Could you check a few things on this model? Use its own coordinates, in mm. Face numbers are marked on the shaded views. A direction names the side the tool comes from. Give positions to 0.01 mm unless a question says otherwise; leave off trailing zeros. Write each loop counter-clockwise with the first axis right and the second up, starting at its lowest first coordinate (ties: lowest second). Pieces come first, ordered by that corner, then holes. Notation, with made-up numbers: M -11,9 L -7,9 A11 ccw -7,24 Z; hole C -24,64 d9. An arc over 180 degrees is marked long. Answer as a JSON object with one key per item and string values. Group by question number.
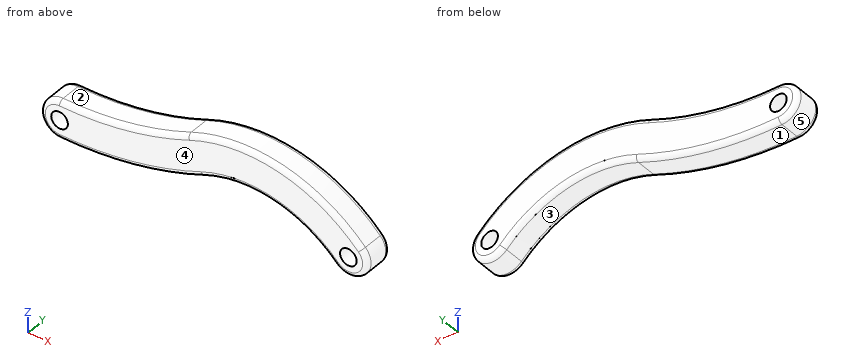
```python
from build123d import *

# Parameters (mm, degrees)
SKETCH1_R           = 1.75
BOSS_EXTRUDE1_DEPTH = 6
FILLET1_R           = 1


with BuildPart() as part:
    # Sketch1 → Boss-Extrude1 (new body)
    with BuildSketch(Plane(origin=(0, 0, 0), x_dir=(1, 0, 0), z_dir=(0, 1, 0))):
        with BuildLine():
            ThreePointArc((-30.4, 4), (-34.4, 0), (-30.4, -4))
            ThreePointArc((-30.4, -4), (-16.617055958, -5.436924168), (-3.426888285, -9.685897488))
            ThreePointArc((-3.426888285, -9.685897488), (15.962258381, -11.93115149), (33.228427125, -2.828427125))
            ThreePointArc((33.228427125, -2.828427125), (33.228427125, 2.828427125), (27.571572875, 2.828427125))
            ThreePointArc((27.571572875, 2.828427125), (14.491142009, -4.067576182), (-0.197605466, -2.366626181))
            ThreePointArc((-0.197605466, -2.366626181), (-14.966930275, 2.391043974), (-30.4, 4))
        make_face()
        with Locations(Location((-30.4, 0, 0), (0, 0, 270))):
            Circle(SKETCH1_R, mode=Mode.SUBTRACT)
        with Locations(Location((30.4, 0, 0), (0, 0, 270))):
            Circle(SKETCH1_R, mode=Mode.SUBTRACT)
    extrude(amount=BOSS_EXTRUDE1_DEPTH)

    # Fillet1
    fillet1_edges = [part.edges().sort_by_distance(p)[0] for p in [
        (-16.617055958, 6, 5.436924168),
        (15.962258381, 6, 11.93115149),
        (33.228427125, 6, -2.828427125),
        (14.491142009, 6, 4.067576182),
        (-14.966930275, 6, -2.391043974),
        (14.491142009, 0, 4.067576182),
        (33.228427125, 0, -2.828427125),
        (15.962258381, 0, 11.93115149),
        (-16.617055958, 0, 5.436924168),
        (-34.4, 0, 0),
        (-14.966930275, 0, -2.391043974),
        (-34.4, 6, 0),
    ]]
    fillet(fillet1_edges, radius=FILLET1_R)


solid = part.part
```
1) We'd pull the mould along X, two halves only. Please class the marked faces 3, 4 and 5: released by +X, released by -X, zero draft, split by the parting line, or undercut.
2) For the marked faces 1 and 2, which set-ups out of +Z, -Z, +X, -X, +Y, -Y let a thin tool reach every point of the face, with its end or its side?
3) If we section it at B-B, the plane z = 0: Give the number of separate pieces and of enclosed holes in the cut face, plus the area to 3 significant figures.
4) If we section it at A-A, the plane y = 3.75: List the corners of the cut face in (x, z) for me, plus the area to 3 significant figures.
5) Please list where these lines run through material, in increasing order: line 1 along Y through (x, z) = (-15, -1.5); line 2 along Z through (x, y) = (-18, 2.25); line 3 along Z through (x, y) = (5.5, 3.25). Write a range as from..to.
6) I'm going to push flat-ended pins straight in: pin 1 (2 mm diameter, centred on x = 30.4, z = 0, fed in from +Y); pin 2 (1 mm diameter, centred on x = 4, y = 5, fed in from -Z); pin 3 (1 mm diameter, centred on x = -10, z = 7, fed in from +Y). Where does each tip first touch, or does it pass through?
Taken from the geometry:
{
 "1": {"face 3": "undercut", "face 4": "zero draft", "face 5": "released by -X"},
 "2": {"face 1": "-Z, +Y, -Y", "face 2": "+Z, -X, +Y, -Y"},
 "3": {"separate pieces": "4", "enclosed holes": "0", "area": "185 mm²"},
 "4": {"outline": "M -30.4,-4 A74.82 ccw -0.2,2.37 A25 cw 27.57,-2.83 A4 ccw 33.23,2.83 A33 ccw -3.43,9.69 A66.82 cw -30.4,4 A4 ccw Z; hole C -30.4,0 d3.5; hole C 30.4,0 d3.5", "area": "545 mm²"},
 "5": {"line 1": "0.01..5.99", "line 2": "-2.97..5.16", "line 3": "4.1..12.2"},
 "6": {"pin 1": "through", "pin 2": "z = 3.66", "pin 3": "y = 5.95"}
}
